Design review of the part shown in the three views and the two pictorial views. Dimensions are in mm from the part's minimum x, y and z. A direction names the side the tool comes from. Round coordinates to 2 decimals unless told otherwise and drop trailing zeros. Order: outer loops, then holes, each group sorted by start corner. A loop starts at its lowest first (then second) coordinate and runs counter-clockwise, first axis right, second up. Notation, with made-up numbers: (-28, 61.5) - (-21, 61.5) arc R11 cw to (-21, 71.5) - close; hole circle Ø10 at (79.5, 79.25). An arc over 180 degrees is marked (long way). One line per item, written item: value.
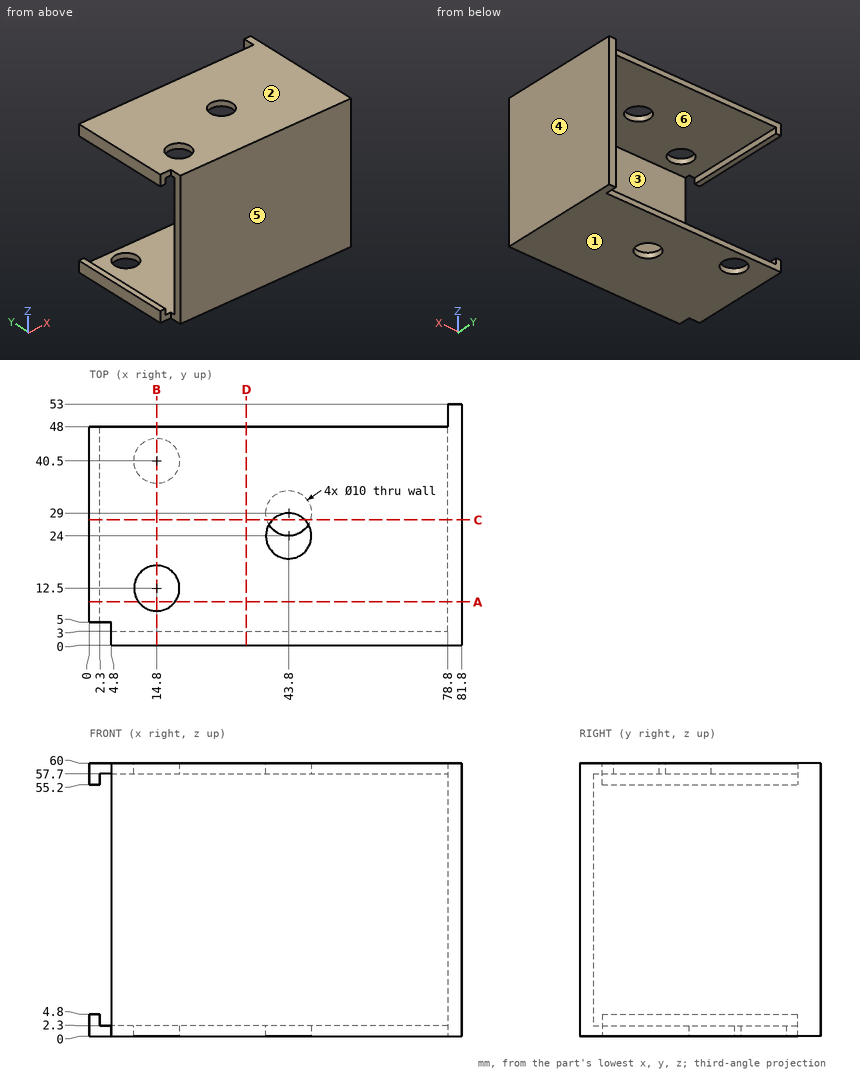
Item 1: Take a section at A-A (y = 9.5). Write out the cut boundary in (x, z).
Returned:
outline: (0, 0) - (81.8, 0) - (81.8, 60) - (18.8, 60) - (18.8, 57.7) - (78.8, 57.7) - (78.8, 2.3) - (2.3, 2.3) - (2.3, 4.8) - (0, 4.8) - close; (0, 55.2) - (2.3, 55.2) - (2.3, 57.7) - (10.8, 57.7) - (10.8, 60) - (0, 60) - close
Item 2: For P1, Ø1, axis at y = 17.5, z = 41, coming from the -X side; P2, Ø3, axis at x = 64, z = 41.5, coming from the +Y side; P3, Ø5.5, axis at x = 2, z = 58, coming from the -Y side, all flat-tipped, find the tip position at first contact; note any pin that passes through.
Returned:
P1: x = 78.8
P2: y = 3
P3: y = 5
Item 3: Machinability: for the marked faces 5 and 6, which of the approach directions +Z, -Z, +X, -X, +Y, -Y give a long, thin tool a straight path to every point of the face, cutting with its end or side? Answer none if there is none.
Returned:
face 5: +Z, -Z, +X, -X, -Y
face 6: +Y
Item 4: The part is to be moulded in two halves that separate along Z. For the marked faces 1, 2, 3 and 4, say which applies: +Z half, -Z half, draft (parallel to the pull), parting line (faces both ways), or undercut.
Returned:
face 1: -Z half
face 2: +Z half
face 3: undercut
face 4: draft
Item 5: Take a section at D-D (x = 34.5). Write out the cut boundary in (y, z).
Returned:
outline: (0, 0) - (48, 0) - (48, 2.3) - (3, 2.3) - (3, 57.7) - (48, 57.7) - (48, 60) - (0, 60) - close
Item 6: Wall thickness on line 1 (Z direction, x = 20, y = 21.5); line 2 (Y direction, x = 14.8, z = 0.9); line 3 (Y direction, x = 59.5, z = 10): over which ranges is each line inside the solid? List them lowest first.
Returned:
line 1: 0 to 2.3, 57.7 to 60
line 2: 0 to 35.5, 45.5 to 48
line 3: 0 to 3
Item 7: Take a section at B-B (x = 14.8). Write out the cut boundary in (y, z).
Returned:
outline: (0, 0) - (35.5, 0) - (35.5, 2.3) - (3, 2.3) - (3, 57.7) - (7.5, 57.7) - (7.5, 60) - (0, 60) - close; (17.5, 57.7) - (48, 57.7) - (48, 60) - (17.5, 60) - close; (45.5, 0) - (48, 0) - (48, 2.3) - (45.5, 2.3) - close
Item 8: Take a section at C-C (y = 27.5). Write out the cut boundary in (x, z).
Returned:
outline: (0, 0) - (39.03, 0) - (39.03, 2.3) - (2.3, 2.3) - (2.3, 4.8) - (0, 4.8) - close; (0, 55.2) - (2.3, 55.2) - (2.3, 57.7) - (40.23, 57.7) - (40.23, 60) - (0, 60) - close; (47.37, 57.7) - (78.8, 57.7) - (78.8, 2.3) - (48.57, 2.3) - (48.57, 0) - (81.8, 0) - (81.8, 60) - (47.37, 60) - close
